from build123d import *

# Parameters (mm, degrees)
F0_W     = 88.9
F0_H     = 38.1
F1_DEPTH = 6.35
F2_T     = -2.54
F4_DEPTH = 2.54


with BuildPart() as f1:
    # F0 (on Top) → F1 (new body)
    with BuildSketch(Plane.XY):
        Rectangle(F0_W, F0_H)
    extrude(amount=F1_DEPTH)

    # F2
    f2_openings = [f1.faces().sort_by_distance(p)[0] for p in [
        (0, 0, 6.35),
    ]]
    offset(amount=F2_T, openings=f2_openings)

    # F3 (on face) → F4 (join)
    with BuildSketch(Plane(origin=(0, 0, 0), x_dir=(1, 0, 0), z_dir=(0, 0, -1))):
        with BuildLine():
            Line((-44.45, -9.525), (-44.45, 9.525))
            ThreePointArc((-44.45, 9.525), (-53.975, 0), (-44.45, -9.525))
        make_face()
    extrude(amount=-F4_DEPTH)


solid = f1.part
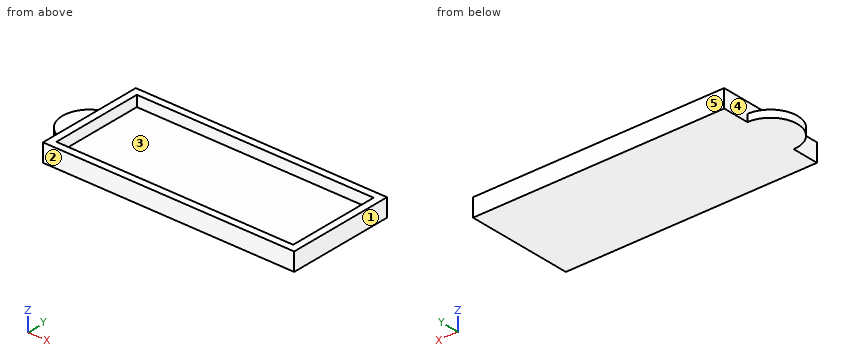
CAD build for the part. Positions are in the model's coordinates, mm. Face numbers are marked on the shaded views. A direction names the side the tool comes from. Coordinates: 2 decimals unless noted, no trailing zeros. Loops run counter-clockwise (first coordinate to the right, second up) from the corner with the lowest first, then second, coordinate; pieces in that order, holes last. Notation, with made-up numbers: (-2.5, 46.5) - (53.5, 46.5) arc R31 cw to (53.5, 79.5) - close; hole circle Ø1 at (23, 19.25). An arc over 180 degrees is marked (long way). Use one line per item in the form item = value. Start each with the question number.
1) Band-saw the part on B-B (y = 14). Give the cut face in (x, z), and give its area (3 significant figures).
2) Tool access for the marked faces 4 and 5: list every direction of +Z, -Z, +X, -X, +Y, -Y with a clear straight run to the whole face (end or side of a thin tool).
3) Drill centre lines: L1, parallel to X at y = -9, z = 3; L2, parallel to Y at x = 11.5, z = 3; L3, parallel to Z at x = -29, y = 2. Where is each one in solid material? Low to high. Write a range as from..to.
4) Two-plate mould, pull along Y, no slides. Class the marked faces 1, 2 and 3: +Y half, -Y half, draft (parallel to the pull), parting line (faces both ways), or undercut.
5) Flat gauge pins, fed straight in: pin 1 (1 mm diameter, centred on y = 7, z = 5.5, fed in from -X); pin 2 (10 mm diameter, centred on x = 2.5, y = 2, fed in from +Z); pin 3 (3 mm diameter, centred on y = 1, z = 1, fed in from -X) (3 decimals). Where does each tip first touch, or does it go through?
6) Band-saw the part on C-C (x = -36). Give the cut face in (y, z).
7) Band-saw the part on D-D (y = 0). Give the cut face in (x, z) (3 decimals).
8) Band-saw the part on A-A (z = 5.5). Give the cut face in (x, y), and give its area (3 significant figures).
Check values:
q1.outline = (-44.45, 0) - (44.45, 0) - (44.45, 6.35) - (41.91, 6.35) - (41.91, 2.54) - (-41.91, 2.54) - (-41.91, 6.35) - (-44.45, 6.35) - close
q1.area = 245 mm2
q2.face_4 = +Z, -X
q2.face_5 = +Z, -Z, +X, -X, +Y
q3.L1 = -44.45..-41.91, 41.91..44.45
q3.L2 = -19.05..-16.51, 16.51..19.05
q3.L3 = 0..2.54
q4.face_1 = draft
q4.face_2 = -Y half
q4.face_3 = undercut
q5.pin_1 = -44.45
q5.pin_2 = 2.54
q5.pin_3 = -53.975
q6.outline = (-19.05, 0) - (19.05, 0) - (19.05, 6.35) - (16.51, 6.35) - (16.51, 2.54) - (-16.51, 2.54) - (-16.51, 6.35) - (-19.05, 6.35) - close
q7.outline = (-53.975, 0) - (44.45, 0) - (44.45, 6.35) - (41.91, 6.35) - (41.91, 2.54) - (-41.91, 2.54) - (-41.91, 6.35) - (-44.45, 6.35) - (-44.45, 2.54) - (-53.975, 2.54) - close
q8.outline = (-44.45, -19.05) - (44.45, -19.05) - (44.45, 19.05) - (-44.45, 19.05) - close; hole (-41.91, -16.51) - (41.91, -16.51) - (41.91, 16.51) - (-41.91, 16.51) - close
q8.area = 619 mm2
